```python
from build123d import *

# Parameters (mm, degrees)
F0_W     = 101.6
F0_H     = 76.2
F1_DEPTH = 127
F3_DEPTH = 76.2
F4_R     = 12.7
F5_R     = 18.977167
F6_DEPTH = 1270


with BuildPart() as f1:
    # F0 (on Front) → F1 (new body)
    with BuildSketch(Plane.XZ):
        with Locations((16.153131, 6.98517)):
            Rectangle(F0_W, F0_H)
    extrude(amount=F1_DEPTH)

    # F2 (on face) → F3 (cut)
    with BuildSketch(Plane.XZ.offset(127)):
        Polygon((12.216878, 45.08517), (-34.646869, 45.08517), (-34.646869, -31.11483), (-17.961076, -31.11483), (8.608649, -17.288411), (29.273987, 0), align=None)
    extrude(amount=-F3_DEPTH, mode=Mode.SUBTRACT)

    # F4
    f4_edges = [f1.edges().sort_by_distance(p)[0] for p in [
        (66.953131, -63.5, 45.08517),
    ]]
    fillet(f4_edges, radius=F4_R)

    # F5 (on face) → F6 (cut)
    with BuildSketch(Plane.XY.offset(45.08517)):
        with Locations((28.853131, -25.4)):
            Circle(F5_R)
    extrude(amount=-F6_DEPTH, mode=Mode.SUBTRACT)


solid = f1.part
```
The model under review builds one solid part; all positions refer to its coordinate system, in mm. A direction names the side the tool comes from. Round coordinates to 2 decimals unless told otherwise and drop trailing zeros. Loops run counter-clockwise (first coordinate to the right, second up) from the corner with the lowest first, then second, coordinate; pieces in that order, holes last. Notation, with made-up numbers: (-40, 8) -> (-3, 8) arc R30 ccw to (-3, 41) -> close; hole circle Ø1 at (86, 24.25). An arc over 180 degrees is marked (long way). Answer as a JSON object with one key per item and string values. Group by question number.
1) Mouldability with a two-part tool opening along Z and no side actions: class faces 4 (the face through (19, -48, 45.085)), 5 (the face through (15, -63, -31.115)), 6 (the face through (18.797, -89.433, -8.765)), 7 (the face through (15, 0, 8)) as released by +Z, released by -Z, zero draft, split by the parting line, or undercut.
2) For pin 1 Ø1 at (y, z) = (-114, -23) entering from -X, flat-tipped, find the tip position at first contact; note if it passes through.
3) For line 1 (X direction, y = -25, z = 3); line 2 (Y direction, x = 1, z = 40.5); line 3 (Y direction, x = 21, z = 18.5), list the stretches that pass through material, from the lowest coordinate up. Write a range as [from, to].
4) We need section A-A on y = -25.4. Write out the cut boundary in (x, z).
5) We need section B-B on x = 37.5. Write out the cut boundary in (y, z).
6) For faces 1 (the face through (-4.862, -89.433, -24.298)), 2 (the face through (46.954, -19.7, 7.519)), 3 (the face through (20.865, -89.433, 22.227)), list the 3-axis set-ups (+Z, -Z, +X, -X, +Y, -Y) from which the entire face can be reached by the end or side of a thin tool; tool diameter is ignored.
7) We need section C-C on z = 21.5. Write out the cut boundary in (x, y).
8) We need section D-D on y = -66. Write out the cut boundary in (x, z), then the cut area to 3 significant figures.
Result set:
{
 "1": {"face 4": "released by +Z", "face 5": "released by -Z", "face 6": "undercut", "face 7": "zero draft"},
 "2": {"pin 1": "x = -3.33"},
 "3": {"line 1": "[-34.65, 9.88], [47.83, 66.95]", "line 2": "[-50.8, 0]", "line 3": "[-50.8, -42.68], [-8.12, 0]"},
 "4": {"outline": "(-34.65, -31.11) -> (9.88, -31.11) -> (9.88, 45.09) -> (-34.65, 45.09) -> close; (47.83, -31.11) -> (66.95, -31.11) -> (66.95, 32.39) arc R12.7 ccw to (54.25, 45.09) -> (47.83, 45.09) -> close"},
 "5": {"outline": "(-127, -31.11) -> (-42.29, -31.11) -> (-42.29, 45.09) -> (-127, 45.09) -> close; (-8.51, -31.11) -> (0, -31.11) -> (0, 45.09) -> (-8.51, 45.09) -> close"},
 "6": {"face 1": "+Z, -X, -Y", "face 2": "+Z, -Z", "face 3": "-X, -Y"},
 "7": {"outline": "(-34.65, -50.8) -> (21.14, -50.8) -> (21.14, -127) -> (66.95, -127) -> (66.95, 0) -> (-34.65, 0) -> close; hole circle Ø37.95 at (28.85, -25.4)"},
 "8": {"outline": "(-17.96, -31.11) -> (66.95, -31.11) -> (66.95, 32.39) arc R12.7 ccw to (54.25, 45.09) -> (12.22, 45.09) -> (29.27, 0) -> (8.61, -17.29) -> close", "area": "3,870 mm²"}
}
